Autodesk Inventor part; units mm, degrees
ref_plane "YZ Plane" through (0, 0, 0) normal (1, 0, 0) x (0, 1, 0)
ref_plane "XZ Plane" through (0, 0, 0) normal (0, 1, 0) x (-1, 0, 0)
ref_plane "XY Plane" through (0, 0, 0) normal (0, 0, 1) x (1, 0, 0)
sketch "Sketch1" plane through (0, 0, 0) normal (0, 1, 0) x (-1, 0, 0)
  line L0 (140, 100) -> (-60, 100)
  line L1 (-60, 100) -> (-60, -100)
  line L2 (-60, -100) -> (140, -100)
  line L3 (140, -100) -> (140, 100)
  line L4 (180, 0) -> (-100, 0) construction
  circle A0 centre (8, 95) radius 2
  circle A1 centre (-8, 95) radius 2
  line L5 (8, 95) -> (-8, 95) construction
  line L6 (0, -140) -> (0, 140) construction
  circle A2 centre (8, -95) radius 2
  circle A3 centre (-8, -95) radius 2
  circle A4 centre (-33, 46) radius 1.85
  circle A5 centre (33, 46) radius 1.85
  line L7 (33, 46) -> (-33, 46) construction
  point P0 (0, 0)
  point P1 (0, 95)
  point P2 (0, 46)
  dimension "d0" = 200
  dimension "d1" = 200
  dimension "d2" = 60
  dimension "d3" = 4
  dimension "d4" = 16
  dimension "d6" = 5
  dimension "d9" = 3.7
  dimension "d10" = 66
  dimension "d11" = 46
extrude "Extrusion1" add sketch "Sketch1" along normal blind 8
sketch "Sketch2" plane through (0, 8, 0) normal (0, 1, 0) x (1, 0, 0)
  line L0 (-122.2, -80) -> (-70, -80)
  line L1 (-70, -80) -> (-70, -40)
  line L2 (-70, -40) -> (-122.2, -40)
  line L3 (-122.2, -40) -> (-122.2, -80)
  line L4 (-140, -100) -> (60, -100) construction
  point P0 (0, 0)
  dimension "d12" = 52.2
  dimension "d13" = 40
  dimension "d14" = 70
  dimension "d15" = 20
extrude "Extrusion2" add sketch "Sketch2" along normal blind 45
chamfer "Chamfer1" distance 39 distance2 40 1 edges at (-96.1, 53, 40) measured on face at (-87.4, 38, 40)
fillet "Fillet1" radius 2 3 edges at (-96.1, 53, 79.9999) (-96.1, 53, 80) (-96.1, 14.0001, 40)
sketch "Sketch3" plane through (-70, 8, 80) normal (1, 0, 0) x (0, 0, -1)
  line L0 (40, 0) -> (0, 0) construction
  line L1 (0, 0) -> (0, 40.2567) construction
  circle A0 centre (8, 6) radius 2
  circle A1 centre (28, 6) radius 2
  circle A2 centre (8, 26) radius 2
  line L2 (8, 6) -> (28, 6) construction
  line L3 (8, 6) -> (8, 26) construction
  point P0 (80, -8)
  dimension "d22" = 4
  dimension "d23" = 20
  dimension "d24" = 20
  dimension "d25" = 8
  dimension "d26" = 6
extrude "Extrusion3" cut sketch "Sketch3" against normal up to surface (52.2 mm away)
sketch "Sketch6" plane through (-70, 8, 80) normal (1, 0, 0) x (0, 0, -1)
  line L0 (0, 0) -> (0, 40.2567)
  arc A0 (3.3962, 41.6887) -> (0, 40.2567) centre (2, 40.2567) ccw
  line L1 (3.3962, 41.6887) -> (39.3962, 6.5887)
  line L2 (11.4963, 33.7911) -> (0, 22)
  point P0 (80, -8)
  dimension "d45" = 22
extrude "Extrusion6" cut sketch "Sketch6" against normal blind 2
sketch "Sketch7" plane through (-122.2, 8, 40) normal (-1, 0, 0) x (0, 0, 1)
  line L0 (28.5037, 33.7911) -> (40, 22)
  line L1 (40, 0) -> (40, 40.2567)
  arc A0 (40, 40.2567) -> (36.6038, 41.6887) centre (38, 40.2567) ccw
  line L2 (36.6038, 41.6887) -> (0.6038, 6.5887)
  point P0 (-40, -8)
extrude "Extrusion7" cut sketch "Sketch7" against normal blind 2
sketch "Sketch4" plane through (0, 0, 0) normal (0, -1, 0) x (1, 0, 0)
  circle A0 centre (-133, 85) radius 1.45
  circle A1 centre (-93, 85) radius 1.45
  line L0 (-133, 85) -> (-93, 85) construction
  line L1 (-113, 85) -> (-113, -85) construction
  line L2 (-133, -85) -> (-93, -85) construction
  circle A2 centre (-133, -85) radius 1.45
  circle A3 centre (-93, -85) radius 1.45
  line L3 (-180, 0) -> (100, 0) construction
  line L4 (-140, 100) -> (60, 100) construction
  point P0 (0, 0)
  dimension "d29" = 2.9
  dimension "d30" = 40
  dimension "d31" = 15
  dimension "d32" = 7
extrude "Extrusion4" cut sketch "Sketch4" against normal up to surface (8 mm away)
fillet "Fillet2" radius 3 4 edges at (60, 4, 100) (-140, 4, 100) (-140, 4, -100) (60, 4, -100)
sketch "Sketch5" plane through (0, 8, 0) normal (0, 1, 0) x (1, 0, 0)
  line L0 (-120, -23.4375) -> (-120, 40)
  line L1 (-120, 40) -> (25, 40)
  line L2 (40, 40) -> (-120, -30) construction
  line L3 (40, 33.4375) -> (40, -30)
  line L4 (40, -30) -> (-105, -30)
  line L5 (-105, -30) -> (40, 33.4375)
  line L6 (-120, -30) -> (-105, -30) construction
  line L7 (40, 40) -> (40, 33.4375) construction
  line L8 (-137, -100) -> (57, -100) construction
  line L9 (60, -97) -> (60, 97) construction
  line L10 (-120, -23.4375) -> (25, 40)
  line L11 (-120, -23.4375) -> (-120, -30) construction
  line L12 (25, 40) -> (40, 40) construction
  point P0 (0, 0)
  dimension "d36" = 160
  dimension "d37" = 70
  dimension "d39" = 15
  dimension "d40" = 70
  dimension "d41" = 20
extrude "Extrusion5" cut sketch "Sketch5" against normal up to surface (8 mm away)
fillet "Fillet3" radius 3 6 edges at (-105, 4, 30) (40, 4, -33.4375) (40, 4, 30) (-120, 4, 23.4375) (-120, 4, -40) (25, 4, -40)
properties part number "Chassis"
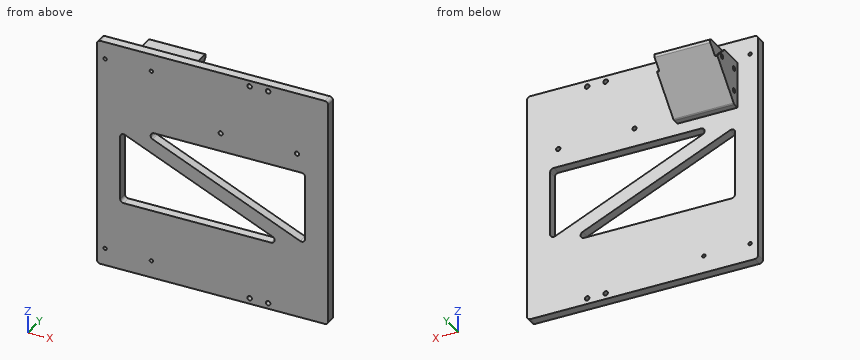
Design review of the part built by this model. Coordinates are the model's own, in mm. Give positions to 0.01 mm unless a question says otherwise; leave off trailing zeros. Loops run counter-clockwise (first coordinate to the right, second up) from the corner with the lowest first, then second, coordinate; pieces in that order, holes last. Notation, with made-up numbers: M 21,70.5 L 60,70.5 A17 ccw 60,94.5 Z; hole C -28.75,55.5 d3. An arc over 180 degrees is marked long. Return JSON: item names as keys, results as strings. Group by question number.
Item 1: For probe 1 along Z at (x, y) = (-133, 3); probe 2 along X at (y, z) = (4, -85); probe 3 along Z at (x, y) = (-8, 5), list the stretches that pass through material, from the lowest coordinate up.
Item 2: We need section D-D (z = 36). Give the boundary of the cut face in (x, y).
Item 3: Insertion check: pin 1 Ø5 at (x, z) = (-118.5, 52.5) entering from -Y; pin 2 Ø5 at (x, z) = (-92, -64.5) entering from +Y. Each pin has a flat end and moves straight along its axis. Give the tip position at first contact, or say it passes through.
Item 4: We need section B-B (z = -17). Give the boundary of the cut face in (x, y).
Item 5: We need section C-C (x = 22). Give the boundary of the cut face in (y, z).
Item 6: We need section A-A (x = -54.5). Give the boundary of the cut face in (y, z), and give its area (4 significant figures).
Output:
{
 "1": {"probe 1": "z = -100 to -86.45, -83.55 to 83.55, 86.45 to 100", "probe 2": "x = -140 to -134.45, -131.55 to -94.45, -91.55 to 60", "probe 3": "z = -100 to -97, -93 to -40, -25.56 to -12.44, 30 to 93, 97 to 100"},
 "2": {"outline": "M -140,0 L 60,0 L 60,8 L -140,8 Z"},
 "3": {"pin 1": "stops at y = 0", "pin 2": "stops at y = 8"},
 "4": {"outline": "M -140,0 L -120,0 L -120,8 L -140,8 Z; M -27.57,0 L 2.43,0 L 2.43,8 L -27.57,8 Z; M 40,0 L 60,0 L 60,8 L 40,8 Z"},
 "5": {"outline": "M 0,-100 L 8,-100 L 8,-25.56 L 0,-25.56 Z; M 0,30 L 8,30 L 8,100 L 0,100 Z"},
 "6": {"outline": "M 0,-100 L 8,-100 L 8,-40 L 0,-40 Z; M 0,-5.22 L 8,-5.22 L 8,7.91 L 0,7.91 Z; M 0,30 L 8,30 L 8,100 L 0,100 Z", "area": "1,145 mm^2"}
}
